Design review of the part shown in the three views and the two pictorial views. Dimensions are in mm from the part's minimum x, y and z. A direction names the side the tool comes from. Round coordinates to 2 decimals unless told otherwise and drop trailing zeros. Write each loop counter-clockwise with the first axis right and the second up, starting at its lowest first coordinate (ties: lowest second). Pieces come first, ordered by that corner, then holes. Notation, with made-up numbers: (82.5, -36) - (132.5, -36) arc R8 ccw to (132.5, -31) - close; hole circle Ø8 at (45.25, 61.5). An arc over 180 degrees is marked (long way). One line per item, written item: value. Start each with the question number.
Q1. For probe 1 along Y at (x, z) = (42.5, 25) (1 decimal); probe 2 along Y at (x, z) = (30, 14.5); probe 3 along Z at (x, y) = (56, 20), list the stretches that pass through material, from the lowest coordinate up.
Q2. Add section B-B on x = 75. Write out the cut boundary in (y, z) (1 decimal).
Q3. Add section A-A on z = 34. Write out the cut boundary in (x, y) (1 decimal).
Q4. Add section D-D on y = 10.25. Write out the cut boundary in (x, z), and give its area (3 significant figures).
Q5. Add section C-C on y = 15.5. Write out the cut boundary in (x, z), and give its area (3 significant figures).
Q6. Tool access review of the marked faces 1, 2 and 3: name each direction out of +Z, -Z, +X, -X, +Y, -Y from which nothing blocks a thin tool from reaching the whole face with its end or side.
Q7. Clearance check with flat-ended pins moving along their axes: pin 1 Ø5 at (x, z) = (32.5, 74) entering from +Y (1 decimal); pin 2 Ø8 at (y, z) = (8, 14.5) entering from -X; pin 3 Ø4 at (x, z) = (21.5, 39) entering from -Y. State where each tip first meets the part, or that it passes through.
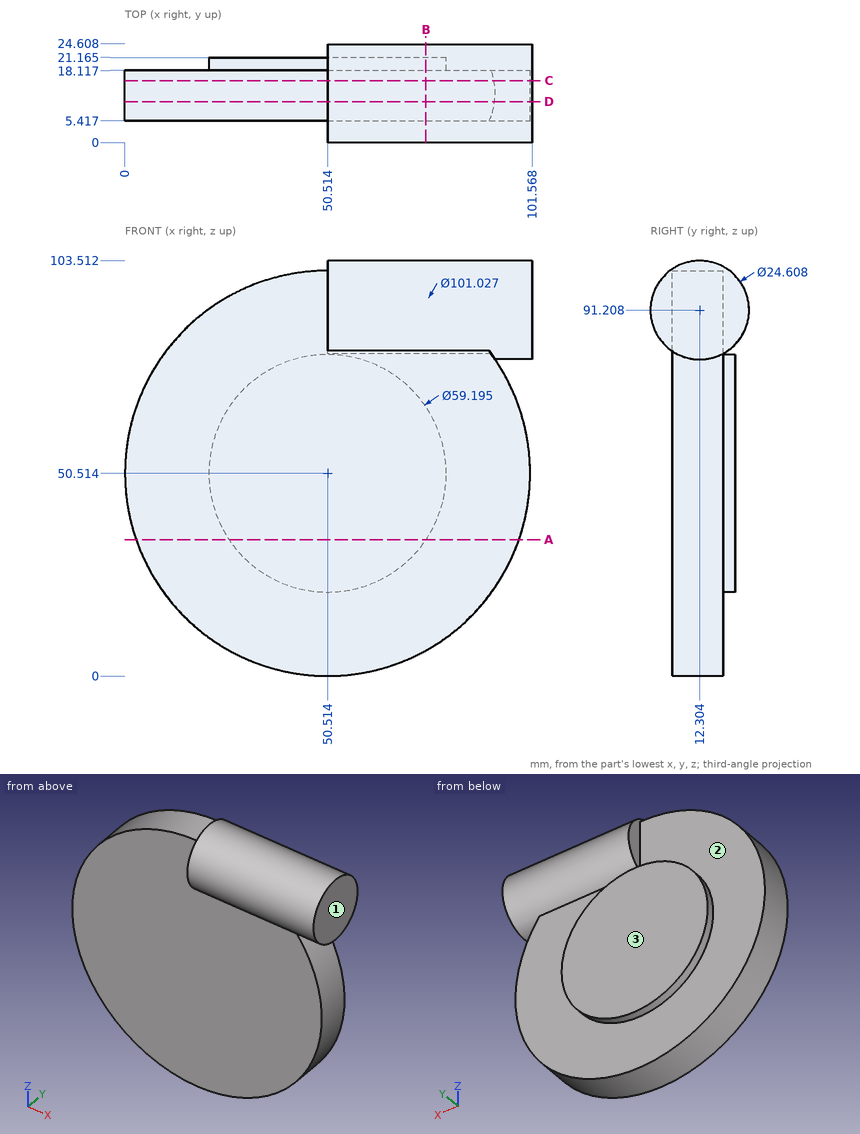
Result set:
1. probe 1: y = 5.4 to 21.2
1. probe 2: y = 5.42 to 18.12
1. probe 3: z = 21.43 to 79.6, 81.61 to 100.81
2. outline: (5.4, 6.3) - (18.1, 6.3) - (18.1, 33.9) - (21.2, 33.9) - (21.2, 67.1) - (18.1, 67.1) - (18.1, 80.4) arc R12.3 ccw (long way) to (5.4, 81) - close
3. outline: (2.8, 5.4) - (98.3, 5.4) - (98.3, 18.1) - (75.1, 18.1) - (75.1, 21.2) - (26, 21.2) - (26, 18.1) - (2.8, 18.1) - close
4. outline: (50.51, 101.03) arc R50.51 ccw (long way) to (92.18, 79.08) - (101.57, 79.08) - (101.57, 103.34) - (50.51, 103.34) - close
4. area: 8,610 mm^2
5. outline: (50.51, 101.03) arc R50.51 ccw (long way) to (92, 79.33) - (101.57, 79.33) - (101.57, 103.09) - (50.51, 103.09) - close
5. area: 8,600 mm^2
6. face 1: +Z, -Z, +X, +Y, -Y
6. face 2: +Y
6. face 3: -Z, +X, -X, +Y
7. pin 1: stops at y = 21.2
7. pin 2: stops at x = 11.44
7. pin 3: stops at y = 5.42
